Check sheet for the modelled part. Datum: model origin and axes. Units: mm. A direction names the side the tool comes from. Give positions to 0.01 mm unless a question says otherwise; leave off trailing zeros. Order: outer loops, then holes, each group sorted by start corner. A loop starts at its lowest first (then second) coordinate and runs counter-clockwise, first axis right, second up.
Item 1: Gauge pin test, flat ends, axial feed: P1, Ø1.6, axis at y = -2.5, z = -5, coming from the +X side; P2, Ø1, axis at y = -2, z = -5, coming from the -X side. Record the tip position at first contact, or that the pin passes through.
Item 2: Sectioned sample at A-A on z = 5. Record the boundary of the cut face in (x, y) (3 decimals), and give its area (3 significant figures).
Item 3: Material ranges on line 1 along X through (y, z) = (-1.3, 5) (3 decimals); line 2 along X through (y, z) = (-1.65, 6.25); line 3 along Z through (x, y) = (35, -1.4) (3 decimals), recorded low to high.
Item 4: Release check for a two-part mould opening along X. For faces 1 (the flat face through (5, -2, -2.8)), 2 (the flat face through (30, -3, -4)), 3 (the flat face through (0, -3, 4)) record: released by +X, released by -X, zero draft, split by the parting line, or undercut.
Item 5: Sectioned sample at B-B on x = 33.5. Record the boundary of the cut face in (y, z), and give its area (3 significant figures).
Item 6: Sectioned sample at C-C on y = -0.75. Record the boundary of the cut face in (x, z) (3 decimals).
Item 7: Sectioned sample at D-D on x = 25. Record the boundary of the cut face in (y, z).
Item 8: Access from +Z, -Z, +X, -X, +Y, -Y to the whole of each face (thin tool, end or side, straight path). Record for faces 4 (the flat face through (25, -2, -2.8)), 5 (the flat face through (20, -5, 2)), 6 (the flat face through (10, -3, -4)).
from build123d import *

# Parameters (mm, degrees)
ESQUISSE1_W                = 40
ESQUISSE1_H                = 5
BOSS_EXTRU_1_DEPTH         = 10
ESQUISSE2_R                = 3.125
ENL_V_MAT_EXTRU_1_DEPTH    = 6
ESQUISSE3_W                = 40
ESQUISSE3_H                = 5
BOSS_EXTRU_2_DEPTH         = 6
CONG_1_R                   = 7
ESQUISSE5_W                = 10
ESQUISSE5_H                = 5
ENL_V_MAT_EXTRU_3_DEPTH    = 3.2
R_P_TITION_LIN_AIRE1_COUNT = 2
R_P_TITION_LIN_AIRE1_PITCH = 20


with BuildPart() as part:
    # Esquisse1 → Boss.-Extru.1 (new body)
    with BuildSketch(Plane.XY):
        with Locations((20, -2.5)):
            Rectangle(ESQUISSE1_W, ESQUISSE1_H)
    extrude(amount=BOSS_EXTRU_1_DEPTH)

    # Esquisse2 → Enlèv. mat.-Extru.1 (cut, through all)
    with BuildSketch(Plane(origin=(0, 0, 0), x_dir=(1, 0, 0), z_dir=(0, 1, 0))):
        with Locations((35, -5)):
            Circle(ESQUISSE2_R)
    extrude(amount=-ENL_V_MAT_EXTRU_1_DEPTH, mode=Mode.SUBTRACT)

    # Esquisse3 → Boss.-Extru.2 (add)
    with BuildSketch(Plane(origin=(0, 0, 0), x_dir=(-1, 0, 0), z_dir=(0, 0, -1))):
        with Locations((-20, -2.5)):
            Rectangle(ESQUISSE3_W, ESQUISSE3_H)
    extrude(amount=BOSS_EXTRU_2_DEPTH)

    # Congé1
    cong_1_edges = [part.edges().sort_by_distance(p)[0] for p in [
        (40, -2.5, -6),
    ]]
    fillet(cong_1_edges, radius=CONG_1_R)

    # Esquisse5 → Enlèv. mat.-Extru.3 (cut)
    with BuildSketch(Plane(origin=(0, 0, -6), x_dir=(-1, 0, 0), z_dir=(0, 0, -1))):
        with Locations((-5, -2.5)):
            Rectangle(ESQUISSE5_W, ESQUISSE5_H)
    enl_v_mat_extru_3 = extrude(amount=-ENL_V_MAT_EXTRU_3_DEPTH, mode=Mode.SUBTRACT)

    # Répétition linéaire1: Enlèv. mat.-Extru.3 ×2
    with Locations(*[(i * R_P_TITION_LIN_AIRE1_PITCH, 0, 0) for i in range(1, R_P_TITION_LIN_AIRE1_COUNT)]):
        add(enl_v_mat_extru_3, mode=Mode.SUBTRACT)


solid = part.part
Report:
1. P1: stops at x = 37.69
1. P2: stops at x = 10
2. outline: (0, -5) - (31.875, -5) - (31.875, 0) - (0, 0) - close; (38.125, -5) - (40, -5) - (40, 0) - (38.125, 0) - close
2. area: 169 mm2
3. line 1: x = 0 to 31.875, 38.125 to 40
3. line 2: x = 0 to 32.14, 37.86 to 40
3. line 3: z = -5.708 to 1.875, 8.125 to 10
4. face 1: zero draft
4. face 2: undercut
4. face 3: released by -X
5. outline: (-5, -5.98) - (0, -5.98) - (0, 2.26) - (-5, 2.26) - close; (-5, 7.74) - (0, 7.74) - (0, 10) - (-5, 10) - close
5. area: 52.5 mm2
6. outline: (0, -2.8) - (10, -2.8) - (10, -6) - (20, -6) - (20, -2.8) - (30, -2.8) - (30, -6) - (33, -6) arc R7 ccw to (40, 1) - (40, 10) - (0, 10) - close; hole circle Ø6.25 at (35, 5)
7. outline: (-5, -2.8) - (0, -2.8) - (0, 10) - (-5, 10) - close
8. face 4: -Z, +Y, -Y
8. face 5: +Z, -Z, +X, -X, -Y
8. face 6: -Z, -X, +Y, -Y
